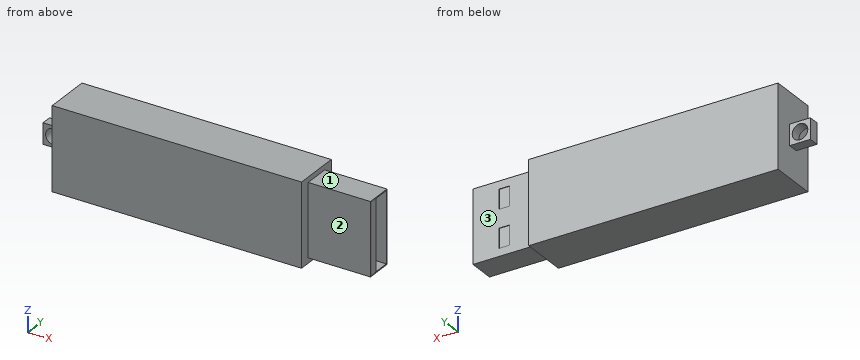
Autodesk Inventor part; units mm, degrees
ref_plane "YZ Plane" through (0, 0, 0) normal (1, 0, 0) x (0, 1, 0)
ref_plane "XZ Plane" through (0, 0, 0) normal (0, 1, 0) x (-1, 0, 0)
ref_plane "XY Plane" through (0, 0, 0) normal (0, 0, 1) x (1, 0, 0)
sketch "Sketch1" plane through (0, 0, 0) normal (0, 0, 1) x (1, 0, 0)
  line L0 (0, 6.3) -> (0, -6.3)
  line L1 (-33.6012, 0) -> (33.607, 0)
  line L2 (-24, 4.5) -> (24, 4.5)
  line L3 (24, 4.5) -> (24, -4.5)
  line L4 (24, -4.5) -> (-24, -4.5)
  line L5 (-24, -4.5) -> (-24, 4.5)
  dimension "d0" = 48
  dimension "d1" = 9
extrude "Legoblokje" add sketch "Sketch1" along normal mid plane 16
sketch "Sketch3" plane through (24, -4.5, 8) normal (1, 0, 0) x (0, 0, -1)
  line L0 (0, 9) -> (0, 0)
  line L1 (0, 0) -> (16, 0)
  line L2 (16, 0) -> (16, 9)
  line L3 (0, 9) -> (16, 9)
  line L4 (1, 7) -> (15, 7)
  line L5 (15, 7) -> (15, 2)
  line L6 (15, 2) -> (1, 2)
  line L7 (1, 2) -> (1, 7)
  point P0 (8, 4.5)
  dimension "d28" = 1
  dimension "d29" = 2
  dimension "d30" = 2
  dimension "d31" = 1
  dimension "d67" = 5
extrude "USB" add sketch "Sketch3" along normal blind 12 contours L4 L5 L6 L7
sketch "Sketch4" plane through (36, -4.5, 8) normal (1, 0, 0) x (0, 0, -1)
  line L0 (15, 7) -> (15, 2)
  line L1 (1, 7) -> (15, 7)
  line L2 (1, 2) -> (1, 7)
  line L3 (15, 2) -> (1, 2)
  line L4 (1.2, 3.7) -> (14.8, 3.7)
  line L5 (14.8, 3.7) -> (14.8, 2.2)
  line L6 (14.8, 2.2) -> (1.2, 2.2)
  line L7 (1.2, 2.2) -> (1.2, 3.7)
  line L8 (1.2, 3.7) -> (14.8, 3.7)
  line L9 (14.8, 3.7) -> (14.8, 6.8)
  line L10 (14.8, 6.8) -> (1.2, 6.8)
  line L11 (1.2, 6.8) -> (1.2, 3.7)
  point P0 (8, 4.5)
  dimension "d34" = 0.2
  dimension "d35" = 0.2
  dimension "d36" = 0.2
  dimension "d37" = 1.5
  dimension "d38" = 0.2
extrude "Afwerking USB" cut sketch "Sketch4" against normal blind 12 contours L11 L10 L9 L4
sketch "Sketch5" plane through (36, -4.5, 8) normal (1, 0, 0) x (0, 0, -1)
  line L0 (15, 2) -> (1, 2)
  line L1 (1.2, 3.7) -> (14.8, 3.7)
  line L2 (14.8, 3.7) -> (14.8, 2.2)
  line L3 (14.8, 2.2) -> (1.2, 2.2)
  line L4 (1.2, 2.2) -> (1.2, 3.7)
  point P0 (8, 4.5)
  dimension "d41" = 0.2
extrude "Afwerking" cut sketch "Sketch5" against normal blind 0.01
sketch "Sketch6" plane through (24, 2.5, 7) normal (0, 1, 0) x (1, 0, 0)
  line L0 (0, 14) -> (12, 14)
  line L1 (0, 0) -> (0, 14)
  line L2 (0, 0) -> (12, 0)
  line L3 (5, 12.5) -> (7, 12.5)
  line L4 (7, 12.5) -> (7, 8.75)
  line L5 (7, 8.75) -> (5, 8.75)
  line L6 (5, 8.75) -> (5, 12.5)
  line L7 (5, 5.25) -> (7, 5.25)
  line L8 (7, 5.25) -> (7, 1.5)
  line L9 (7, 1.5) -> (5, 1.5)
  line L10 (5, 1.5) -> (5, 5.25)
  point P0 (-24, 7)
  dimension "d44" = 5
  dimension "d45" = 5
  dimension "d46" = 1.5
  dimension "d47" = 1.5
  dimension "d48" = 3.5
  dimension "d49" = 2
  dimension "d50" = 2
  dimension "d51" = 3.75
  dimension "d52" = 3.75
extrude "Afwerking bovenkant" cut sketch "Sketch6" against normal blind 0.1
sketch "Sketch7" plane through (-24, -4.5, 8) normal (-1, 0, 0) x (0, 0, 1)
  line L0 (-10, 5.5) -> (-6, 5.5)
  line L1 (-6, 5.5) -> (-6, 3.5)
  line L2 (-6, 3.5) -> (-10, 3.5)
  line L3 (-10, 3.5) -> (-10, 5.5)
  point P0 (-8, 4.5)
  dimension "d55" = 1
  dimension "d56" = 1
  dimension "d57" = 2
  dimension "d58" = 2
extrude "Achterkant afwerking" add sketch "Sketch7" along normal blind 4
sketch "Sketch8" plane through (-24, 1, 2) normal (0, 1, 0) x (1, 0, 0)
  circle A0 centre (-2, 2) radius 1.5
  point P0 (24, 2)
  dimension "d61" = 3
extrude "afwerking gat" cut sketch "Sketch8" against normal through all
properties part number "USB_Stick"
The model under review builds one solid part; all positions refer to its coordinate system, in mm. Face numbers are marked on the shaded views. A direction names the side the tool comes from. Give positions to 0.01 mm unless a question says otherwise; leave off trailing zeros. Write each loop counter-clockwise with the first axis right and the second up, starting at its lowest first coordinate (ties: lowest second). Pieces come first, ordered by that corner, then holes.
1. For P1, Ø0.6, axis at x = -25.5, y = 0, coming from the +Z side; P2, Ø0.9, axis at y = 1, z = -2, coming from the +X side; P3, Ø6, axis at x = 31.5, z = 3, coming from the -Y side; P4, Ø2.5, axis at x = -26, z = 0, coming from the +Y side, all flat-tipped, find the tip position at first contact; note any pin that passes through.
2. Add section A-A, the plane x = -26. Write out the cut boundary in (y, z).
3. Wall thickness on L1, parallel to X at y = -0.45, z = 0; L2, parallel to Z at x = -26, y = -0.5; L3, parallel to X at y = -3.5, z = 1.75: over which ranges is each line inside the solid? List them lowest first.
4. Add section C-C, the plane x = 32. Write out the cut boundary in (y, z), plus the area to 3 significant figures.
5. Add section D-D, the plane y = -3.5. Write out the cut boundary in (x, z), plus the area to 3 significant figures.
6. Tool access review of the marked faces 1, 2 and 3: name each direction out of +Z, -Z, +X, -X, +Y, -Y from which nothing blocks a thin tool from reaching the whole face with its end or side.
Worked answers:
1. P1: stops at z = 2
1. P2: stops at x = 24
1. P3: stops at y = -2.5
1. P4: passes through
2. outline: (-1, -2) - (1, -2) - (1, -1.5) - (-1, -1.5) - close; (-1, 1.5) - (1, 1.5) - (1, 2) - (-1, 2) - close
3. L1: x = -28 to -27.5, -24.5 to 24
3. L2: z = -2 to -1.5, 1.5 to 2
3. L3: x = -24 to 24
4. outline: (-2.5, -7) - (2.5, -7) - (2.5, 7) - (-2.5, 7) - close; hole (-0.8, -6.8) - (2.3, -6.8) - (2.3, 6.8) - (-0.8, 6.8) - close
4. area: 27.8 mm2
5. outline: (-24, -8) - (24, -8) - (24, 8) - (-24, 8) - close
5. area: 768 mm2
6. face 1: +Z, +X, +Y, -Y
6. face 2: +Z, -Z, +X, -Y
6. face 3: +Z, -Z, +X, +Y
